Source: CAD feature listing. Evaluate the final solid. Frame: model axes, mm. Face numbers are marked on the shaded views. Coordinates: 2 decimals unless noted, no trailing zeros. Order: outer loops, then holes, each group sorted by start corner. A loop starts at its lowest first (then second) coordinate and runs counter-clockwise, first axis right, second up. Notation, with made-up numbers: (-18.5, 71.25) -> (-6.5, 71.25) arc R28 ccw to (-6.5, 103.25) -> close; hole circle Ø6 at (-2, -40). An arc over 180 degrees is marked (long way). Write each question's results on one line, items separated by ' | '. Start each with the question number.
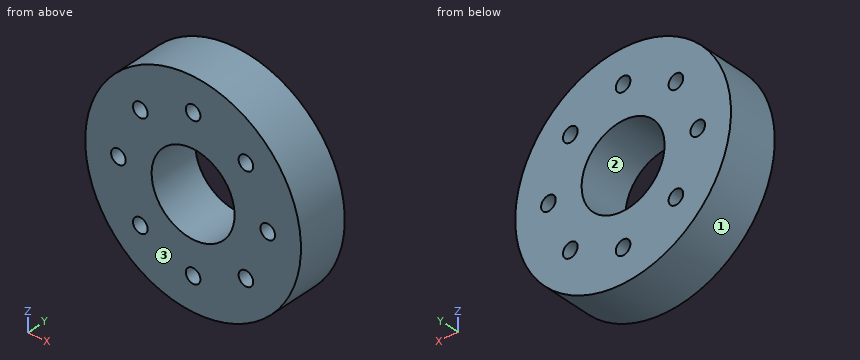
from build123d import *

# Parameters (mm, degrees)
SKETCH1_R           = 32.5
BOSS_EXTRUDE1_DEPTH = 15
SKETCH2_R           = 2.2
CUT_EXTRUDE1_DEPTH  = 49.347699015
SKETCH3_R           = 12.5
CUT_EXTRUDE2_DEPTH  = 49.347699015


with BuildPart() as part:
    # Sketch1 → Boss-Extrude1 (new body)
    with BuildSketch(Plane(origin=(0, 0, 0), x_dir=(1, 0, 0), z_dir=(0, 1, 0))):
        with Locations(Location((0, 0, 0), (0, 0, 270))):
            Circle(SKETCH1_R)
    extrude(amount=BOSS_EXTRUDE1_DEPTH)

    # Sketch2 → Cut-Extrude1 (cut, through all)
    with BuildSketch(Plane(origin=(0, 15, 0), x_dir=(1, 0, 0), z_dir=(0, 1, 0))):
        with Locations(Location((0, 22.5, 0), (0, 0, 270))):
            Circle(SKETCH2_R)
        with Locations(Location((15.909902577, 15.909902577, 0), (0, 0, 270))):
            Circle(SKETCH2_R)
        with Locations(Location((22.5, 0, 0), (0, 0, 270))):
            Circle(SKETCH2_R)
        with Locations(Location((15.909902577, -15.909902577, 0), (0, 0, 270))):
            Circle(SKETCH2_R)
        with Locations(Location((0, -22.5, 0), (0, 0, 270))):
            Circle(SKETCH2_R)
        with Locations(Location((-15.909902577, -15.909902577, 0), (0, 0, 270))):
            Circle(SKETCH2_R)
        with Locations(Location((-22.5, 0, 0), (0, 0, 270))):
            Circle(SKETCH2_R)
        with Locations(Location((-15.909902577, 15.909902577, 0), (0, 0, 270))):
            Circle(SKETCH2_R)
    extrude(amount=-CUT_EXTRUDE1_DEPTH, mode=Mode.SUBTRACT)

    # Sketch3 → Cut-Extrude2 (cut, through all)
    with BuildSketch(Plane(origin=(0, 15, 0), x_dir=(1, 0, 0), z_dir=(0, 1, 0))):
        with Locations(Location((0, 0, 0), (0, 0, 270))):
            Circle(SKETCH3_R)
    extrude(amount=-CUT_EXTRUDE2_DEPTH, mode=Mode.SUBTRACT)


solid = part.part
(1) Draft query along X for the marked faces 1, 2 and 3. Return one class per face: released by +X, released by -X, zero draft, split by the parting line, or undercut.
(2) First-contact query: P1, Ø4, axis at x = -22.5, z = 0, coming from the +Y side; P2, Ø3, axis at x = 2.5, y = 12, coming from the -Z side; P3, Ø1, axis at x = 9, y = 3.5, coming from the -Z side; P4, Ø8, axis at x = -8.5, y = 4.5, coming from the -Z side. Flat tips, straight axial feed; report the tip coordinate or a pass-through.
(3) Section D-D on x = 14.5. Return the cut outline in (y, z).
(4) Section B-B on x = 0. Return the cut outline in (y, z).
(5) Section C-C on z = -15. Return the cut outline in (x, y).
(6) Section A-A on z = 0. Return the cut outline in (x, y), then the cut area to 3 significant figures.
(7) Line query: L1, parallel to X at y = 9.5, z = 0; L2, parallel to Z at x = 17, y = 7.5; L3, parallel to X at y = 10.75, z = -14.5. Output: solid intervals per line, ascending.
Results list:
1) face 1: split by the parting line | face 2: undercut | face 3: zero draft
2) P1: passes through | P2: stops at z = -32.48 | P3: stops at z = -31.37 | P4: stops at z = -32.19
3) outline: (0, -29.09) -> (15, -29.09) -> (15, -17.6) -> (0, -17.6) -> close; (0, -14.22) -> (15, -14.22) -> (15, 14.22) -> (0, 14.22) -> close; (0, 17.6) -> (15, 17.6) -> (15, 29.09) -> (0, 29.09) -> close
4) outline: (0, -32.5) -> (15, -32.5) -> (15, -24.7) -> (0, -24.7) -> close; (0, -20.3) -> (15, -20.3) -> (15, -12.5) -> (0, -12.5) -> close; (0, 12.5) -> (15, 12.5) -> (15, 20.3) -> (0, 20.3) -> close; (0, 24.7) -> (15, 24.7) -> (15, 32.5) -> (0, 32.5) -> close
5) outline: (-28.83, 0) -> (-17.91, 0) -> (-17.91, 15) -> (-28.83, 15) -> close; (-13.91, 0) -> (13.91, 0) -> (13.91, 15) -> (-13.91, 15) -> close; (17.91, 0) -> (28.83, 0) -> (28.83, 15) -> (17.91, 15) -> close
6) outline: (-32.5, 0) -> (-24.7, 0) -> (-24.7, 15) -> (-32.5, 15) -> close; (-20.3, 0) -> (-12.5, 0) -> (-12.5, 15) -> (-20.3, 15) -> close; (12.5, 0) -> (20.3, 0) -> (20.3, 15) -> (12.5, 15) -> close; (24.7, 0) -> (32.5, 0) -> (32.5, 15) -> (24.7, 15) -> close | area: 468 mm²
7) L1: x = -32.5 to -24.7, -20.3 to -12.5, 12.5 to 20.3, 24.7 to 32.5 | L2: z = -27.7 to -17.82, -14 to 14, 17.82 to 27.7 | L3: x = -29.09 to -17.6, -14.22 to 14.22, 17.6 to 29.09
